Build history of the part. All positions in model axes, mm. A direction names the side the tool comes from. Give positions to 0.01 mm unless a question says otherwise; leave off trailing zeros. Loops run counter-clockwise (first coordinate to the right, second up) from the corner with the lowest first, then second, coordinate; pieces in that order, holes last. Notation, with made-up numbers: M 36.5,67 L 59.5,67 A9 ccw 59.5,73 Z; hole C 40,-8 d7. An arc over 180 degrees is marked long. Answer as a JSON object with one key per item and string values. Group by question number.
1. Slice it at C-C (x = -66). List the corners of the cut face in (y, z), then the cut area to 3 significant figures.
2. Slice it at D-D (y = -32.5). List the corners of the cut face in (x, z).
3. Slice it at A-A (x = -15). List the corners of the cut face in (y, z).
4. Drill centre lines: line 1 along X through (y, z) = (-24.5, 119); line 2 along X through (y, z) = (-28, 132); line 3 along X through (y, z) = (-12, 19.5). Where is each one in solid material? Low to high. Write a range as [from, to].
5. Drop flat-ended pins along their axis: pin 1 Ø4.5 at (x, z) = (-2, 123) entering from -Y; pin 2 Ø6 at (x, y) = (-17.5, -65) entering from +Z; pin 3 Ø15 at (x, y) = (3.5, -62) entering from -Z. Give the stop position or say it passes through.
6. 3-axis set-ups, long thin cutter, end or side, ignore diameter. For faces 4 (the face through (-133.728, -30, 120)), 5 (the face through (-25, -30, 128)), 6 (the face through (0, -65, 147.73)): which of +Z, -Z, +X, -X, +Y, -Y reach the whole face in a straight line?
7. Slice it at B-B (z = 74.5). List the corners of the cut face in (x, y), then the cut area to 3 significant figures.
8. Mould opens along Z. For faces 1 (the face through (0, -5.178, 123)), 2 (the face through (-92, 0, 38)), 3 (the face through (0, -25, 115.845)) say: released by +Z, released by -Z, zero draft, split by the parting line, or undercut.
from build123d import *

# Parameters (mm, degrees)
BOSS_EXTRUDE1_DEPTH      = 150
BOSS_EXTRUDE1_DEPTH_BACK = 150
CUT_EXTRUDE3_DEPTH       = 375.5
CUT_EXTRUDE6_DEPTH       = 329
SKETCH9_W                = 271.336979698
SKETCH9_H                = 135.998838498
CUT_EXTRUDE9_DEPTH       = 30
SKETCH10_W               = 95.8
SKETCH10_H               = 62.546807737
CUT_EXTRUDE11_DEPTH      = 30
SKETCH11_W               = 102.1
SKETCH11_H               = 157.042427203
BOSS_EXTRUDE2_DEPTH      = 30
FILLET4_R                = 8
FILLET5_R                = 8
FILLET6_R                = 8
FILLET7_R                = 8
FILLET8_R                = 8
FILLET9_R                = 8
BOSS_EXTRUDE3_DEPTH      = 12
BOSS_EXTRUDE4_START      = -15
BOSS_EXTRUDE4_DEPTH      = 15
SKETCH17_W               = 271.728058528
SKETCH17_H               = 26.824087215
BOSS_EXTRUDE5_DEPTH      = 54
CUT_EXTRUDE14_DEPTH      = 21
CUT_EXTRUDE14_DEPTH_BACK = 21
SKETCH18_W               = 50
SKETCH18_H               = 40
CUT_EXTRUDE15_START      = -349
CUT_EXTRUDE15_DEPTH      = 349


with BuildPart() as part:
    # Sketch2 → Boss-Extrude1 (new, two sides: drawn at the far end of the back side and taken through both)
    with BuildSketch(Plane(origin=(0, 0, 0), x_dir=(0, 0, -1), z_dir=(1, 0, 0)).offset(-BOSS_EXTRUDE1_DEPTH_BACK)):
        with BuildLine():
            Line((47.021092325, 21.603077895), (47.021092325, -52.096922105))
            Line((47.021092325, -52.096922105), (-7.482950192, -79.488697318))
            Line((-7.482950192, -79.488697318), (-154.582950192, -79.488697318))
            ThreePointArc((-154.582950192, -79.488697318), (-141.2900932, -24.98088898), (-110.021334878, 21.603077895))
            Line((-110.021334878, 21.603077895), (47.021092325, 21.603077895))
        make_face()
    extrude(amount=BOSS_EXTRUDE1_DEPTH + BOSS_EXTRUDE1_DEPTH_BACK)

    # Sketch6 → Cut-Extrude3 (cut)
    with BuildSketch(Plane(origin=(150, 0, 0), x_dir=(0, 0, -1), z_dir=(1, 0, 0))):
        Polygon((47.021092325, -52.096922105), (47.021092325, -48.996922105), (-6.950510533, -77.430419395), (-6.23203774, -78.860033625), align=None)
    extrude(amount=-CUT_EXTRUDE3_DEPTH, mode=Mode.SUBTRACT)

    # Sketch8 → Cut-Extrude6 (cut)
    with BuildSketch(Plane(origin=(150, 0, 0), x_dir=(0, 0, -1), z_dir=(1, 0, 0))):
        with BuildLine():
            Line((-18.049462918, -65.128698573), (-139.30133294, -65.128698573))
            ThreePointArc((-139.30133294, -65.128698573), (-127.051990379, -22.399103161), (-99.746787758, 12.676395797))
            Line((-99.746787758, 12.676395797), (32.391473071, 12.676395797))
            Line((32.391473071, 12.676395797), (32.391473071, -41.004772665))
            Line((32.391473071, -41.004772665), (-18.049462918, -65.128698573))
        make_face()
    extrude(amount=-CUT_EXTRUDE6_DEPTH, mode=Mode.SUBTRACT)

    # Sketch9 → Cut-Extrude9 (cut)
    with BuildSketch(Plane.XZ.offset(79.488697318)):
        with Locations((1.940431321, 79.730726135)):
            Rectangle(SKETCH9_W, SKETCH9_H)
    extrude(amount=-CUT_EXTRUDE9_DEPTH, mode=Mode.SUBTRACT)

    # Sketch10 → Cut-Extrude11 (cut)
    with BuildSketch(Plane(origin=(0, 21.603077895, 0), x_dir=(1, 0, 0), z_dir=(0, 1, 0))):
        with Locations((0, -78.74793101)):
            Rectangle(SKETCH10_W, SKETCH10_H)
    extrude(amount=-CUT_EXTRUDE11_DEPTH, mode=Mode.SUBTRACT)

    # Sketch11 → Boss-Extrude2 (add)
    with BuildSketch(Plane(origin=(0, 0, 0), x_dir=(1, 0, 0), z_dir=(0, 1, 0))):
        with Locations((-98.95, -31.500121276)):
            Rectangle(SKETCH11_W, SKETCH11_H)
        with Locations((98.95, -31.500121276)):
            Rectangle(SKETCH11_W, SKETCH11_H)
    extrude(amount=BOSS_EXTRUDE2_DEPTH)

    # Fillet4
    fillet4_edges = [part.edges().sort_by_distance(p)[0] for p in [
        (-98.95, 30, 110.021334878),
    ]]
    fillet(fillet4_edges, radius=FILLET4_R)

    # Fillet5
    fillet5_edges = [part.edges().sort_by_distance(p)[0] for p in [
        (98.95, 30, 110.021334878),
    ]]
    fillet(fillet5_edges, radius=FILLET5_R)

    # Fillet6
    # the kernel refuses this fillet: 8 mm, written as the material it adds along each edge
    with BuildSketch(Plane(origin=(-150, 21.603077895, 110.021334878), x_dir=(0, -0.7256761067447404, 0.6880364729429655), z_dir=(1, 0, 0))) as fillet6_piece_1:
        with BuildLine():
            CenterArc((2.744889422, -7.999720666), FILLET6_R, 90.478801773, 31.768597775)
            Line((-1.523719625, -1.233704348), (-1.950580529, -0.557102717))
            ThreePointArc((-1.950580529, -0.557102717), (-0.838466066, 0.307444001), (-0.550429178, 0.580540885))
            Line((-0.550429178, 0.580540885), (0.006685256, 0.799972067))
            ThreePointArc((0.006685256, 0.799972067), (1.33901843, 0.794405102), (2.671351604, 0.799972067))
            Line((2.671351604, 0.799972067), (2.67803686, 0))
        make_face()
    extrude(amount=102.1)
    # the kernel refuses this fillet: 8 mm, written as the material it takes off along each edge

    # Fillet7
    # the kernel refuses this fillet: 8 mm, written as the material it adds along each edge
    with BuildSketch(Plane(origin=(47.9, 21.603077895, 110.021334878), x_dir=(0, 0.9969460846976341, -0.07809292033249748), z_dir=(1, 0, 0))) as fillet7_piece_1:
        with BuildLine():
            CenterArc((2.900642421, 7.944571871), FILLET7_R, 231.482877932, 31.768597775)
            Line((-2.081345425, 1.685195137), (-2.579544209, 1.059257463))
            ThreePointArc((-2.579544209, 1.059257463), (-1.540564119, 0.225193287), (-0.508590223, -0.617524077))
            Line((-0.508590223, -0.617524077), (0.062474336, -0.797556868))
            ThreePointArc((0.062474336, -0.797556868), (0.458184274, -0.766560061), (1.866538405, -0.794457187))
            Line((1.866538405, -0.794457187), (1.960547861, 0))
        make_face()
    extrude(amount=102.1)
    # the kernel refuses this fillet: 8 mm, written as the material it takes off along each edge

    # Fillet8
    fillet8_edges = [part.edges().sort_by_distance(p)[0] for p in [
        (98.95, 30, -47.021092325),
    ]]
    fillet(fillet8_edges, radius=FILLET8_R)

    # Fillet9
    fillet9_edges = [part.edges().sort_by_distance(p)[0] for p in [
        (-98.95, 30, -47.021092325),
    ]]
    fillet(fillet9_edges, radius=FILLET9_R)

    # Sketch13 → Boss-Extrude3 (add)
    with BuildSketch(Plane(origin=(150, 0, 0), x_dir=(0, 0, -1), z_dir=(1, 0, 0))):
        with BuildLine():
            Line((-139.30133294, -65.128698573), (-18.049462918, -65.128698573))
            Line((-18.049462918, -65.128698573), (32.391473071, -41.004772665))
            Line((32.391473071, -41.004772665), (32.391473071, 0))
            Line((32.391473071, 0), (-110.021334878, 0))
            Line((-110.021334878, 0), (-110.021334878, 2.512453321))
            ThreePointArc((-110.021334878, 2.512453321), (-130.12762054, -28.941917181), (-139.30133294, -65.128698573))
        make_face()
    extrude(amount=-BOSS_EXTRUDE3_DEPTH)

    # Sketch15 → Boss-Extrude4 (add)
    with BuildSketch(Plane.ZY.offset(150).offset(BOSS_EXTRUDE4_START)):
        with BuildLine():
            Line((-32.391473071, 0), (-32.391473071, -41.004772665))
            Line((-32.391473071, -41.004772665), (18.049462918, -65.128698573))
            Line((18.049462918, -65.128698573), (139.30133294, -65.128698573))
            ThreePointArc((139.30133294, -65.128698573), (130.12762054, -28.941917181), (110.021334878, 2.512453321))
            Line((110.021334878, 2.512453321), (110.021334878, 0))
            Line((110.021334878, 0), (-32.391473071, 0))
        make_face()
    extrude(amount=BOSS_EXTRUDE4_DEPTH)

    # Sketch17 → Boss-Extrude5 (add)
    with BuildSketch(Plane.XZ.offset(49.488697318)):
        with Locations((2.135970736, 123.433378486)):
            Rectangle(SKETCH17_W, SKETCH17_H)
    extrude(amount=-BOSS_EXTRUDE5_DEPTH)

    # Sketch18 → Cut-Extrude14 (cut, two sides: drawn at the far end of the back side and taken through both)
    with BuildSketch(Plane.XY.offset(136.845422093).offset(-CUT_EXTRUDE14_DEPTH_BACK)):
        with Locations((0, -25.17833284)):
            Rectangle(SKETCH18_W, SKETCH18_H)
    extrude(amount=CUT_EXTRUDE14_DEPTH + CUT_EXTRUDE14_DEPTH_BACK, mode=Mode.SUBTRACT)

    # Sketch20 → Cut-Extrude15 (cut)
    with BuildSketch(Plane(origin=(150, 0, 0), x_dir=(0, 0, -1), z_dir=(1, 0, 0)).offset(CUT_EXTRUDE15_START)):
        with BuildLine():
            Line((-136.845422093, 4.511302682), (-124.344519516, 4.511302682))
            ThreePointArc((-124.344519516, 4.511302682), (-130.970660544, -5.3695664), (-136.845422093, -15.714830799))
            Line((-136.845422093, -15.714830799), (-136.845422093, 4.511302682))
        make_face()
    extrude(amount=CUT_EXTRUDE15_DEPTH, mode=Mode.SUBTRACT)


solid = part.part
Established:
{
 "1": {"outline": "M -79.49,7.48 L -78.86,6.23 L -77.43,6.95 L -49,-47.02 L 22,-47.02 A8 ccw 30,-39.02 L 30,102.02 A8 ccw 23.56,109.87 A8 cw 19.66,111.86 A160.24 ccw -79.49,154.58 L -79.49,147.73 L -49.49,147.73 L -49.49,110.02 L 0,110.02 L 0,-32.39 L -41,-32.39 L -62.11,11.73 L -79.49,11.73 Z", "area": "8,050 mm^2"},
 "2": {"outline": "M -150,-47.02 L 150,-47.02 L 150,144.38 L 25,144.38 L 25,115.85 L -25,115.85 L -25,144.38 L -150,144.38 Z; hole M -135,-32.39 L 138,-32.39 L 138,110.02 L -133.73,110.02 L -133.73,131.6 L -135,131.6 Z"},
 "3": {"outline": "M -79.49,7.48 L -78.86,6.23 L -77.43,6.95 L -49,-47.02 L 21.6,-47.02 L 21.6,47.47 L 12.68,47.47 L 12.68,-32.39 L -41,-32.39 L -62.11,11.73 L -79.49,11.73 Z; M -79.49,147.73 L -49.49,147.73 L -49.49,110.02 L 21.6,110.02 A160.24 ccw -5.18,130.85 L -5.18,115.85 L -45.18,115.85 L -45.18,148.62 A160.24 ccw -79.49,154.58 Z"},
 "4": {"line 1": "x = [-150, -135], [-133.73, -25], [25, 150]", "line 2": "x = [-150, -25], [25, 150]", "line 3": "x = [-150, -135], [138, 150]"},
 "5": {"pin 1": "stops at y = -49.49", "pin 2": "stops at z = 153.44", "pin 3": "stops at z = -36.58"},
 "6": {"face 4": "none", "face 5": "+Z", "face 6": "-Y"},
 "7": {"outline": "M -150,-79.49 L -133.73,-79.49 L -133.73,-65.13 L -135,-65.13 L -135,0 L -47.9,0 L -47.9,30 L -150,30 Z; M 47.9,0 L 138,0 L 138,-65.13 L 137.61,-65.13 L 137.61,-79.49 L 150,-79.49 L 150,30 L 47.9,30 Z", "area": "8,300 mm^2"},
 "8": {"face 1": "zero draft", "face 2": "undercut", "face 3": "released by +Z"}
}
